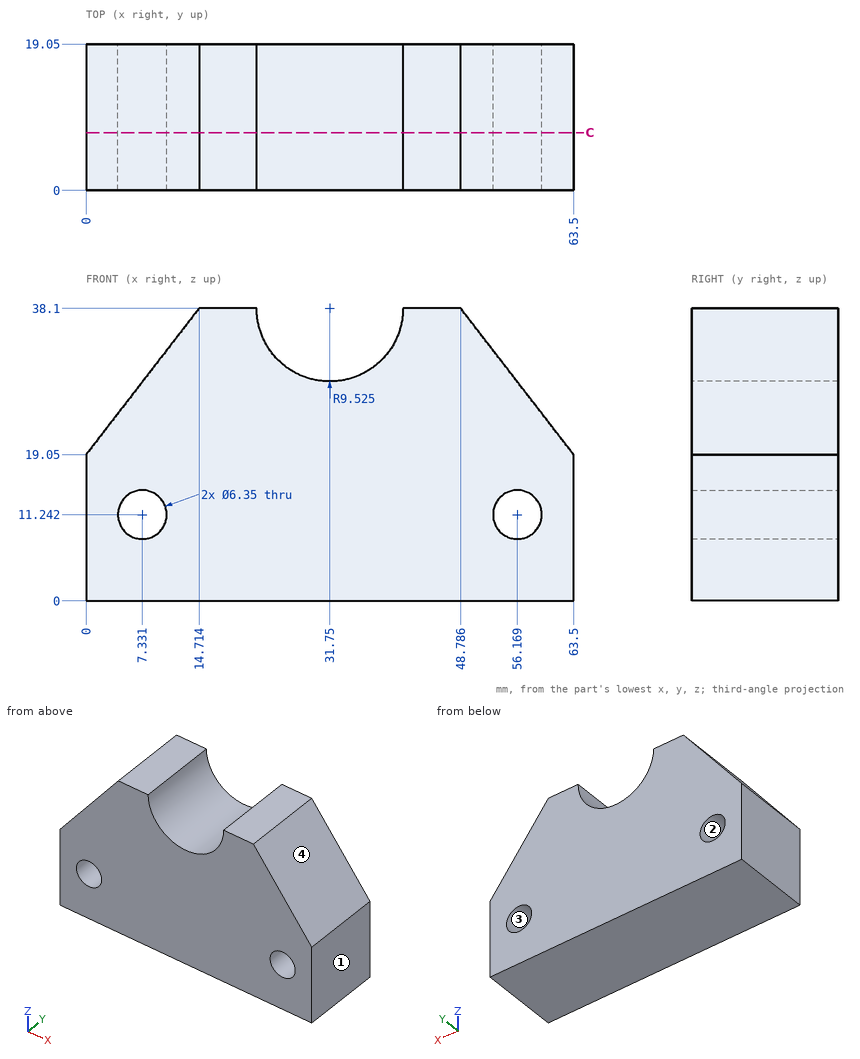
Print and shaded views of the part. All mm, measured from the part's lowest x, y and z. Round coordinates to 2 decimals unless told otherwise and drop trailing zeros. Write each question's results on one line, items separated by ' | '. Start each with the question number.
Item 1: Wall check: L1, parallel to X at y = 3.75, z = 10.5 (1 decimal); L2, parallel to X at y = 1, z = 8.5 (1 decimal); L3, parallel to Z at x = 10, y = 9.5 (1 decimal). Give the ranges that are in metal, low to high. Write a range as [from, to].
Item 2: Saw through at C-C (y = 7.5). State how many separate pieces and enclosed holes the cut face has, and give its area (3 significant figures).
Item 3: Mould opens along Z. For the marked faces 1, 2, 3 and 4 say: pulls with the +Z half, pulls with the -Z half, needs draft (parallel to the pull), parting line crosses it, or undercut.
Results are:
1) L1: x = [0, 4.2], [10.4, 53.1], [59.3, 63.5] | L2: x = [0, 5.7], [8.9, 54.6], [57.8, 63.5] | L3: z = [0, 9.5], [13, 32]
2) separate pieces: 1 | enclosed holes: 2 | area: 1,930 mm²
3) face 1: needs draft | face 2: undercut | face 3: undercut | face 4: pulls with the +Z half
